Design review of the part built by this model. Coordinates are the model's own, in mm. Coordinates: 2 decimals unless noted, no trailing zeros. Loops run counter-clockwise (first coordinate to the right, second up) from the corner with the lowest first, then second, coordinate; pieces in that order, holes last. Notation, with made-up numbers: (43, 4.5) -> (64, 4.5) arc R20 cw to (64, 38.5) -> close; hole circle Ø11 at (51.5, -21.75). An arc over 180 degrees is marked (long way). One line per item, written item: value. Start each with the question number.
1. Insertion check: pin 1 (1.5 mm diameter, centred on x = -56, z = 1, fed in from -Y). The pin has a flat end and moves straight along its axis. Give the tip position at first contact, or say it passes through.
2. Add section B-B on x = -119. Write out the cut boundary in (y, z) (1 decimal).
3. Add section C-C on y = 15. Write out the cut boundary in (x, z) (1 decimal).
4. Add section A-A on z = 0. Write out the cut boundary in (x, y) (3 decimals), plus the area to 3 significant figures.
5. For probe 1 along X at (y, z) = (17, 0) (3 decimals); probe 2 along Y at (x, z) = (-90, 0) (3 decimals); probe 3 along X at (y, z) = (33.5, 2), list the stretches that pass through material, from the lowest coordinate up.
```python
from build123d import *

# Parameters (mm, degrees)
ESBO_O4_R = 4.7625


with BuildPart() as part:
    # Varredura1: sweep along a path in Esboço1
    with BuildLine(Plane.XY) as varredura1_path:
        Line((-200, 157.4625), (0, 157.4625))
        ThreePointArc((0, 157.4625), (12.347852166, 152.347852166), (17.4625, 140))
        Line((17.4625, 140), (17.4625, 0))
        ThreePointArc((17.4625, 0), (12.347852166, -12.347852166), (0, -17.4625))
        Line((0, -17.4625), (-200, -17.4625))
        ThreePointArc((-200, -17.4625), (-212.347852166, -12.347852166), (-217.4625, 0))
        Line((-217.4625, 0), (-217.4625, 140))
        ThreePointArc((-217.4625, 140), (-212.347852166, 152.347852166), (-200, 157.4625))
    # Esboço4 → Varredura1 (sweep)
    with BuildSketch(Plane(origin=(-200, 0, 0), x_dir=(0, 0, -1), z_dir=(1, 0, 0))):
        with Locations((0, 157.4625)):
            Circle(ESBO_O4_R)
    sweep(path=varredura1_path.line)


solid = part.part
```
Worked answers:
1. pin 1: stops at y = -22.22
2. outline: circle Ø9.5 at (-17.5, 0); circle Ø9.5 at (157.5, 0)
3. outline: circle Ø9.5 at (-217.5, 0); circle Ø9.5 at (17.5, 0)
4. outline: (-222.225, 0) arc R22.225 ccw to (-200, -22.225) -> (0, -22.225) arc R22.225 ccw to (22.225, 0) -> (22.225, 140) arc R22.225 ccw to (0, 162.225) -> (-200, 162.225) arc R22.225 ccw to (-222.225, 140) -> close; hole (-212.7, 0) arc R12.7 ccw to (-200, -12.7) -> (0, -12.7) arc R12.7 ccw to (12.7, 0) -> (12.7, 140) arc R12.7 ccw to (0, 152.7) -> (-200, 152.7) arc R12.7 ccw to (-212.7, 140) -> close
4. area: 7,520 mm²
5. probe 1: x = -222.225 to -212.7, 12.7 to 22.225
5. probe 2: y = -22.225 to -12.7, 152.7 to 162.225
5. probe 3: x = -221.78 to -213.14, 13.14 to 21.78
